Geometry check sheet. Reference: the model listing, model coordinates, mm. A direction names the side the tool comes from. Give positions to 0.01 mm unless a question says otherwise; leave off trailing zeros. Loops run counter-clockwise (first coordinate to the right, second up) from the corner with the lowest first, then second, coordinate; pieces in that order, holes last. Notation, with made-up numbers: (-37, -13) -> (-25, -13) arc R24 ccw to (-25, 19) -> close; hole circle Ø4 at (35.25, -4.5). An arc over 180 degrees is marked (long way). Answer in a Markdown table with one row per item. Add a question column.
```python
from build123d import *

# Parameters (mm, degrees)
F0_W      = 2
F0_H      = 9
F0_W_2    = 24
F1_DEPTH  = 22
F3_R      = 20
F4_DEPTH  = 12
F5_R      = 5
F5_R_2    = 4.05
F6_DEPTH  = 50
F7_R      = 2
F8_DEPTH  = 9.001
F9_R      = 11
F10_DEPTH = 2
F11_R     = 1.5
F12_DEPTH = 20
F13_R     = 6
F14_DEPTH = 25
F15_DEPTH = 9


with BuildPart() as f1:
    # F0 (on Front) → F1 (new body, symmetric)
    with BuildSketch(Plane.XZ):
        with BuildLine():
            Line((-16, 51.5), (-16, 60.5))
            ThreePointArc((-16, 60.5), (-28.7279220614, 55.2279220614), (-34, 42.5))
            Line((-34, 42.5), (-34, -30))
            ThreePointArc((-34, -30), (-31.3639610307, -36.3639610307), (-25, -39))
            Line((-25, -39), (-25, -30))
            Line((-25, -30), (-25, 0))
            Line((-25, 0), (-25, 42.5))
            ThreePointArc((-25, 42.5), (-22.3639610307, 48.8639610307), (-16, 51.5))
        make_face()
        with Locations((-15, 56)):
            Rectangle(F0_W, F0_H)
        with Locations((-2, 56)):
            Rectangle(F0_W_2, F0_H)
        Polygon((-25, -30), (-25, -39), (29, -39), (29, -30), (-11.5, -30), align=None)
    extrude(amount=F1_DEPTH, both=True)

    # F0 (on Front) → F2 (revolve)
    with BuildSketch(Plane.XZ):
        Polygon((34, 64), (10, 64), (10, 60.5), (10, 51.5), (10, 48), (34, 48), align=None)
    revolve(axis=Axis((10, 0, 55.4929765165), (0, 0, -1)))

    # F3 (on face) → F4 (cut)
    with BuildSketch(Plane.XY.offset(64)):
        with Locations((10, 0)):
            Circle(F3_R)
    extrude(amount=-F4_DEPTH, mode=Mode.SUBTRACT)

    # F5 (on face) → F6 (cut)
    with BuildSketch(Plane.XY.offset(52)):
        with Locations((10, 0)):
            Circle(F5_R)
        with Locations((20, 0)):
            Circle(F5_R_2)
    extrude(amount=-F6_DEPTH, mode=Mode.SUBTRACT)

    # F7 (on face) → F8 (cut, through all)
    with BuildSketch(Plane.YZ.offset(-25)):
        with Locations((14, -22.5)):
            Circle(F7_R)
        with Locations((14, 32.5)):
            Circle(F7_R)
        with Locations((0, 32.5)):
            Circle(F7_R)
        with Locations((-14, -22.5)):
            Circle(F7_R)
        with Locations((-14, 32.5)):
            Circle(F7_R)
    extrude(amount=-F8_DEPTH, mode=Mode.SUBTRACT)

    # F9 (on face) → F10 (cut)
    with BuildSketch(Plane(origin=(0, 0, -39), x_dir=(1, 0, 0), z_dir=(0, 0, -1))):
        with Locations((10, 0)):
            Circle(F9_R)
    extrude(amount=-F10_DEPTH, mode=Mode.SUBTRACT)

    # F11 (on face) → F12 (cut)
    with BuildSketch(Plane(origin=(0, 0, -39), x_dir=(1, 0, 0), z_dir=(0, 0, -1))):
        with Locations((-3.5, -13.5)):
            Circle(F11_R)
        with Locations((-3.5, 14.5)):
            Circle(F11_R)
        with Locations((24.5, -13.5)):
            Circle(F11_R)
        with Locations((24.5, 14.5)):
            Circle(F11_R)
        with Locations((52.5, -13.5)):
            Circle(F11_R)
        with Locations((52.5, 14.5)):
            Circle(F11_R)
    extrude(amount=-F12_DEPTH, mode=Mode.SUBTRACT)

    # F13 (on face) → F14 (cut)
    with BuildSketch(Plane(origin=(0, 0, -39), x_dir=(1, 0, 0), z_dir=(0, 0, -1))):
        with Locations((10, 0)):
            Circle(F13_R)
    extrude(amount=-F14_DEPTH, mode=Mode.SUBTRACT)

    # F0 (on Front) → F15 (join, symmetric)
    with BuildSketch(Plane.XZ):
        Polygon((-11.5, -30), (-25, 0), (-25, -30), align=None)
    extrude(amount=F15_DEPTH, both=True)


solid = f1.part
```
1. Release check for a two-part mould opening along X. For faces 1 (the face through (23, -14.57, -34.56)), 2 (the face through (29, 0, -35)), 3 (the face through (-29.437, -14.26, -20.517)) record: released by +X, released by -X, zero draft, split by the parting line, or undercut.
2. Sectioned sample at A-A (x = 10). Enter the section's corners in (y, z).
3. Material ranges on L1, parallel to Y at x = 24.5, z = -33.75; L2, parallel to Y at x = 10, z = 51; L3, parallel to Z at x = -3, y = -8, recorded low to high. Write a range as from..to.
4. Access from +Z, -Z, +X, -X, +Y, -Y to the whole of each face (thin tool, end or side, straight path). Record for faces 4 (the face through (-21, -9, -21)), 5 (the face through (-14.4, -1.7, 60.5)), 6 (the face through (10, -6, 48)), 7 (the face through (23, 13.43, -34.56)).
5. Sectioned sample at B-B (z = 32.5). Enter the section's corners in (x, y), plus the area to 3 significant figures.
6. Gauge pin test, flat ends, axial feed: pin 1 Ø11 at (x, y) = (10, 0) entering from -Z; pin 2 Ø20 at (x, y) = (4.5, -6.5) entering from +Z; pin 3 Ø5 at (y, z) = (-14, -22.5) entering from +X; pin 4 Ø4.5 at (y, z) = (14, 32.5) entering from -X. Record the tip position at first contact, or that the pin passes through.
7. Sectioned sample at D-D (z = -22.5). Enter the section's corners in (x, y) (3 decimals).
8. Sectioned sample at C-C (x = 19). Enter the section's corners in (y, z), plus the area to 3 significant figures.
Response:
| question | item | result |
|---|---|---|
| 1 | face 1 | undercut |
| 1 | face 2 | released by +X |
| 1 | face 3 | zero draft |
| 2 | outline | (-24, 48) -> (-5, 48) -> (-5, 52) -> (-20, 52) -> (-20, 64) -> (-24, 64) -> close; (-22, -39) -> (-11, -39) -> (-11, -37) -> (-6, -37) -> (-6, -30) -> (-22, -30) -> close; (5, 48) -> (24, 48) -> (24, 64) -> (20, 64) -> (20, 52) -> (5, 52) -> close; (6, -37) -> (11, -37) -> (11, -39) -> (22, -39) -> (22, -30) -> (6, -30) -> close |
| 3 | L1 | y = -22..-16, -13..12, 15..22 |
| 3 | L2 | y = -24..-5, 5..24 |
| 3 | L3 | z = -39..-30, 48..52 |
| 4 | face 4 | +X, -Y |
| 4 | face 5 | +Z, -X |
| 4 | face 6 | +X, +Y, -Y |
| 4 | face 7 | -Z |
| 5 | outline | (-34, -22) -> (-25, -22) -> (-25, -16) -> (-34, -16) -> close; (-34, -12) -> (-25, -12) -> (-25, -2) -> (-34, -2) -> close; (-34, 2) -> (-25, 2) -> (-25, 12) -> (-34, 12) -> close; (-34, 16) -> (-25, 16) -> (-25, 22) -> (-34, 22) -> close |
| 5 | area | 288 mm2 |
| 6 | pin 1 | stops at z = 48 |
| 6 | pin 2 | stops at z = 52 |
| 6 | pin 3 | stops at x = -25 |
| 6 | pin 4 | stops at x = -34 |
| 7 | outline | (-34, -22) -> (-25, -22) -> (-25, -16) -> (-34, -16) -> close; (-34, -12) -> (-25, -12) -> (-25, -9) -> (-14.875, -9) -> (-14.875, 9) -> (-25, 9) -> (-25, 12) -> (-34, 12) -> close; (-34, 16) -> (-25, 16) -> (-25, 22) -> (-34, 22) -> close |
| 8 | outline | (-22.25, 48) -> (-3.92, 48) -> (-3.92, 52) -> (-17.86, 52) -> (-17.86, 64) -> (-22.25, 64) -> close; (-22, -39) -> (-6.32, -39) -> (-6.32, -37) -> (6.32, -37) -> (6.32, -39) -> (22, -39) -> (22, -30) -> (-22, -30) -> close; (3.92, 48) -> (22.25, 48) -> (22.25, 64) -> (17.86, 64) -> (17.86, 52) -> (3.92, 52) -> close |
| 8 | area | 623 mm2 |
